from build123d import *

# Parameters (mm, degrees)
F0_W      = 44.45
F0_H      = 44.45
F1_DEPTH  = 44.45
F4_DEPTH  = 6.35
F5_W      = 17.78
F5_H      = 6.35
F6_DEPTH  = 6.35
F8_DEPTH  = 6.35
F10_DEPTH = 6.35
F11_DEPTH = 6.35
F13_DEPTH = 6.35
F6_FACE_W = 17.78
F6_FACE_H = 6.35
F14_DEPTH = 6.35


with BuildPart() as f1:
    # F0 (on Front) → F1 (new body)
    with BuildSketch(Plane.XZ):
        with Locations((22.225, 22.225)):
            Rectangle(F0_W, F0_H)
    extrude(amount=F1_DEPTH)

    # F3 (on face) → F4 (join)
    with BuildSketch(Plane.YZ.offset(44.45)):
        Polygon((-27.94, 25.4), (-27.94, 6.35), (-16.51, 6.35), (-16.51, 25.4), (-6.35, 25.4), (-6.35, 38.1), (-38.1, 38.1), (-38.1, 25.4), align=None)
    extrude(amount=F4_DEPTH)

    # F5 (on Front) → F6 (join)
    with BuildSketch(Plane.XZ):
        Polygon((25.4, 6.35), (38.1, 6.35), (38.1, 38.1), (6.35, 38.1), (6.35, 19.05), (12.7, 19.05), (6.35, 6.35), (19.05, 6.35), (25.4, 19.05), align=None)
        with Locations((22.225, 28.575)):
            Rectangle(F5_W, F5_H, mode=Mode.SUBTRACT)
    extrude(amount=-F6_DEPTH)

    # F7 (on face) → F8 (join)
    with BuildSketch(Plane.XY.offset(44.45)):
        Polygon((19.05, -6.35), (6.35, -6.35), (6.35, -38.1), (19.05, -38.1), (19.05, -26.1793940588), (25.4, -26.1793940588), (25.4, -38.1), (38.1, -38.1), (38.1, -6.35), (25.4, -6.35), (25.4, -18.5593940588), (19.05, -18.5593940588), align=None)
    extrude(amount=F8_DEPTH)

    # F9 (on face) → F10 (join)
    with BuildSketch(Plane(origin=(0, 0, 0), x_dir=(1, 0, 0), z_dir=(0, 0, -1))):
        Polygon((6.35, 38.1), (6.35, 6.35), (16.51, 6.35), (16.51, 22.225), (27.94, 6.35), (38.1, 6.35), (38.1, 38.1), (27.94, 38.1), (27.94, 22.225), (16.51, 38.1), align=None)
    extrude(amount=F10_DEPTH)

    # F2 (on face) → F11 (join)
    with BuildSketch(Plane.XZ.offset(44.45)):
        Polygon((19.05, 38.1), (6.35, 38.1), (6.35, 6.35), (19.05, 6.35), (19.05, 22.225), (25.4, 6.35), (38.1, 6.35), (31.75, 22.225), (38.1, 38.1), (25.4, 38.1), (19.05, 27.94), align=None)
    extrude(amount=F11_DEPTH)

    # F12 (on face) → F13 (join)
    with BuildSketch(Plane(origin=(0, 0, 0), x_dir=(0, -1, 0), z_dir=(-1, 0, 0))):
        Polygon((6.35, 38.1), (6.35, 6.35), (19.05, 6.35), (19.05, 22.225), (25.4, 6.35), (38.1, 6.35), (31.75, 22.225), (38.1, 38.1), (25.4, 38.1), (19.05, 27.94), (19.05, 38.1), align=None)
    extrude(amount=F13_DEPTH)

    # F5 (on Front) + F6_face (on face) → F14 (join)
    with BuildSketch(Plane.XZ):
        Polygon((25.4, 6.35), (38.1, 6.35), (38.1, 38.1), (6.35, 38.1), (6.35, 19.05), (12.7, 19.05), (6.35, 6.35), (19.05, 6.35), (25.4, 19.05), align=None)
        with Locations((22.225, 28.575)):
            Rectangle(F5_W, F5_H, mode=Mode.SUBTRACT)
    with BuildSketch(Plane(origin=(22.225, 0, 28.575), x_dir=(-1, 0, 0), z_dir=(0, 1, 0))):
        Rectangle(F6_FACE_W, F6_FACE_H)
    extrude(amount=F14_DEPTH, dir=(0, -1, 0))


solid = f1.part
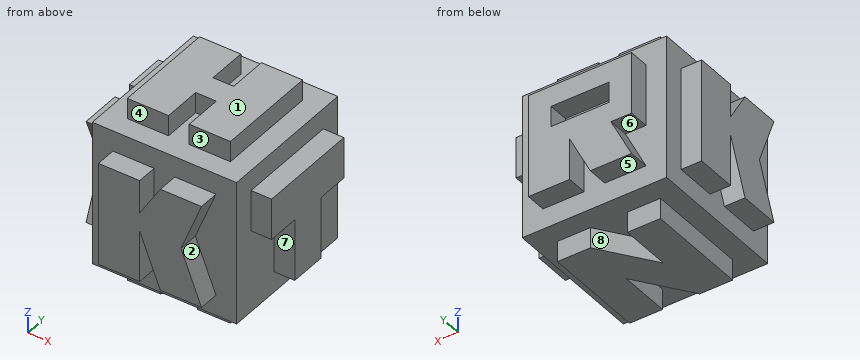
The listing builds one solid part. Answer for the finished solid, in the listing's coordinates (mm). Face numbers are marked on the shaded views. A direction names the side the tool comes from. Round coordinates to 2 decimals unless told otherwise and drop trailing zeros. Order: outer loops, then holes, each group sorted by start corner. A loop starts at its lowest first (then second) coordinate and runs counter-clockwise, first axis right, second up. Notation, with made-up numbers: (34, -8) -> (43, -8) arc R10 cw to (43, 5) -> close; hole circle Ø9 at (-7, 74.25). An arc over 180 degrees is marked (long way). One line per item, written item: value.
Item 1: Find section B-B, the plane y = 2. Give the vertices of the cut face in (x, z) (3 decimals), then the cut area to 3 significant figures.
Taken from the geometry:
outline: (6.35, 6.35) -> (19.05, 6.35) -> (25.4, 19.05) -> (25.4, 6.35) -> (38.1, 6.35) -> (38.1, 38.1) -> (6.35, 38.1) -> (6.35, 19.05) -> (12.7, 19.05) -> close; hole (13.335, 25.4) -> (31.115, 25.4) -> (31.115, 31.75) -> (13.335, 31.75) -> close
area: 815 mm2
Item 2: Straight lines are drawn through the part: L1, parallel to Y at x = 36, z = 21; L2, parallel to Y at x = 27, z = 40; L3, parallel to X at y = -9.5, z = 4. For each, find the intervals that lie inside material, in ascending order.
Taken from the geometry:
L1: y = -44.45 to 6.35
L2: y = -44.45 to 0
L3: x = 0 to 44.45
Item 3: For the marked faces 4, 5, 6, 7 and 8, determine the directions among +Z, -Z, +X, -X, +Y, -Y from which every point of the face is accessible in a straight line to the end or side of a thin tool.
Taken from the geometry:
face 4: +Z, +X, -X, -Y
face 5: -Z, +X, -X, +Y
face 6: -X, +Y
face 7: -Z, +X, -Y
face 8: -Z, +Y
Item 4: For a pull along Z with two mould halves and no side action, classify the marked faces 1, 2 and 3 as released by +Z, released by -Z, zero draft, split by the parting line, or undercut.
Taken from the geometry:
face 1: released by +Z
face 2: undercut
face 3: zero draft
Item 5: Find section D-D, the plane y = -8.5. Give the vertices of the cut face in (x, z).
Taken from the geometry:
outline: (-6.35, 6.35) -> (0, 6.35) -> (0, 0) -> (6.35, 0) -> (6.35, -6.35) -> (16.51, -6.35) -> (16.51, 0) -> (26.39, 0) -> (26.39, -6.35) -> (38.1, -6.35) -> (38.1, 0) -> (44.45, 0) -> (44.45, 25.4) -> (50.8, 25.4) -> (50.8, 38.1) -> (44.45, 38.1) -> (44.45, 44.45) -> (38.1, 44.45) -> (38.1, 50.8) -> (25.4, 50.8) -> (25.4, 44.45) -> (19.05, 44.45) -> (19.05, 50.8) -> (6.35, 50.8) -> (6.35, 44.45) -> (0, 44.45) -> (0, 38.1) -> (-6.35, 38.1) -> close
Item 6: Find section A-A, the plane z = -2. Give the vertices of the cut face in (x, y) (3 decimals).
Taken from the geometry:
outline: (6.35, -38.1) -> (16.51, -38.1) -> (27.94, -22.225) -> (27.94, -38.1) -> (38.1, -38.1) -> (38.1, -6.35) -> (27.94, -6.35) -> (16.51, -22.225) -> (16.51, -6.35) -> (6.35, -6.35) -> close
Item 7: Find section C-C, the plane x = -3. Give the vertices of the cut face in (y, z) (3 decimals).
Taken from the geometry:
outline: (-38.1, 6.35) -> (-25.4, 6.35) -> (-19.05, 22.225) -> (-19.05, 6.35) -> (-6.35, 6.35) -> (-6.35, 38.1) -> (-19.05, 38.1) -> (-19.05, 27.94) -> (-25.4, 38.1) -> (-38.1, 38.1) -> (-31.75, 22.225) -> close
Item 8: Given P1, Ø6, axis at x = 42.5, z = 23, coming from the -Y side; P2, Ø7, axis at y = -10.5, z = -2, coming from the +X side; P3, Ø1.5, axis at x = 42, y = -0.5, coming from the +Z side, each flat-ended and moving along its own axis, determine where each tip first touches the part or whether it passes through.
Taken from the geometry:
P1: stops at y = -44.45
P2: stops at x = 44.45
P3: stops at z = 44.45
